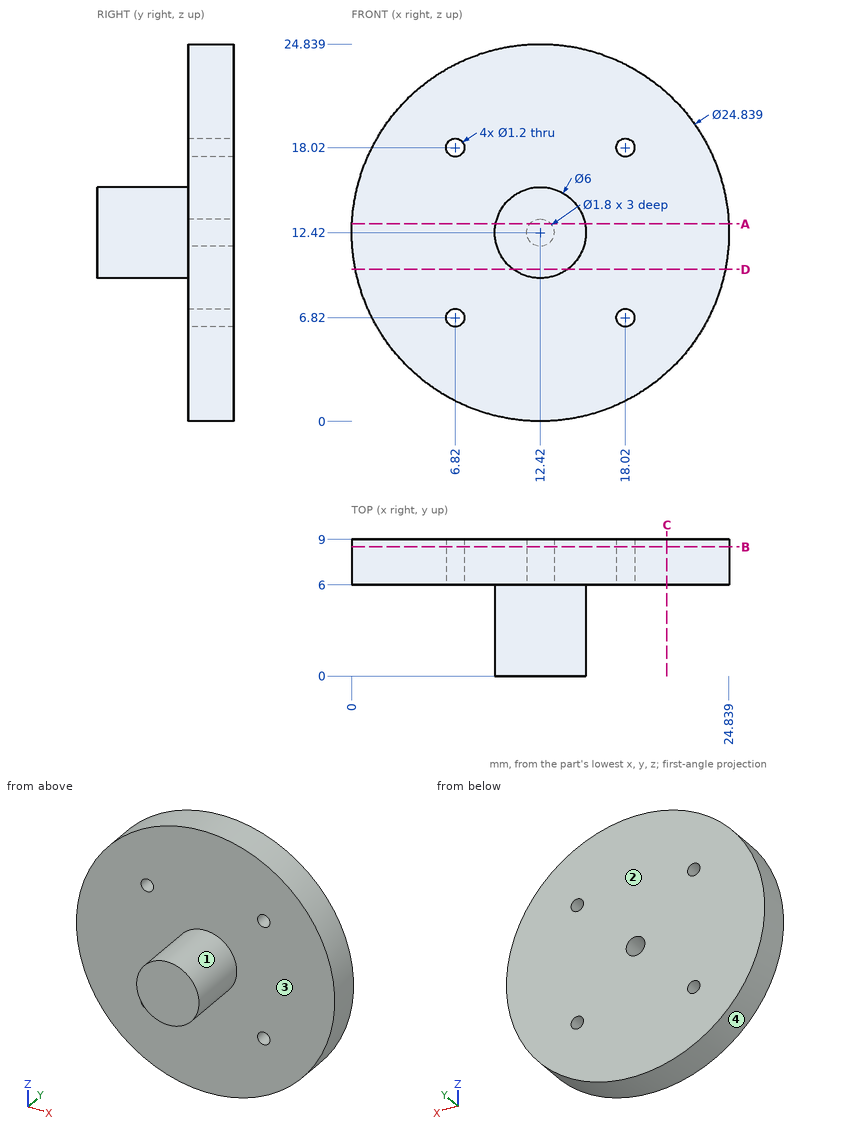
Design review of the part shown in the three views and the two pictorial views. Dimensions are in mm from the part's minimum x, y and z. A direction names the side the tool comes from. Round coordinates to 2 decimals unless told otherwise and drop trailing zeros. Loops run counter-clockwise (first coordinate to the right, second up) from the corner with the lowest first, then second, coordinate; pieces in that order, holes last.
1) The part is to be moulded in two halves that separate along Z. For the marked faces 3 and 4, say which applies: pulls with the +Z half, pulls with the -Z half, needs draft (parallel to the pull), parting line crosses it, or undercut.
Values follow:
face 3: needs draft
face 4: parting line crosses it
2) Consider section D-D on z = 10. State the section outline as (x, y) points.
Values follow:
outline: (0.24, 6) - (10.65, 6) - (10.65, 0) - (14.19, 0) - (14.19, 6) - (24.6, 6) - (24.6, 9) - (0.24, 9) - close
3) Consider section C-C on x = 20.75. State the section outline as (y, z) points.
Values follow:
outline: (6, 3.21) - (9, 3.21) - (9, 21.63) - (6, 21.63) - close
4) Consider section A-A on z = 13. State the section outline as (x, y) points (1 decimal).
Values follow:
outline: (0, 6) - (9.5, 6) - (9.5, 0) - (15.4, 0) - (15.4, 6) - (24.8, 6) - (24.8, 9) - (13.1, 9) - (13.1, 6) - (11.7, 6) - (11.7, 9) - (0, 9) - close
5) Tool access review of the marked faces 1 and 2: name each direction out of +Z, -Z, +X, -X, +Y, -Y from which nothing blocks a thin tool from reaching the whole face with its end or side.
Values follow:
face 1: -Y
face 2: +Z, -Z, +X, -X, +Y
6) Wall thickness on line 1 along Y through (x, z) = (17, 1.75); line 2 along Z through (x, y) = (12.5, 5.75); line 3 along X through (y, z) = (2.25, 12.25) (1 decimal): over which ranges is each line inside the solid? List them lowest first.
Values follow:
line 1: y = 6 to 9
line 2: z = 9.42 to 15.42
line 3: x = 9.4 to 15.4
7) Clearance check with flat-ended pins moving along their axes: P1, Ø1, axis at x = 6.82, z = 18.02, coming from the +Y side; P2, Ø6, axis at x = 15, z = 20, coming from the -Y side; P3, Ø3, axis at x = 10, y = 1, coming from the +Z side (1 decimal); P4, Ø4, axis at x = 15, y = 7, coming from the -Z side. State where each tip first meets the part, or that it passes through.
Values follow:
P1: passes through
P2: stops at y = 6
P3: stops at z = 15.3
P4: stops at z = 0.01
8) Consider section B-B on y = 8.5. State the section outline as (x, z) points.
Values follow:
outline: circle Ø24.84 at (12.42, 12.42); hole circle Ø1.2 at (6.82, 6.82); hole circle Ø1.2 at (6.82, 18.02); hole circle Ø1.8 at (12.42, 12.42); hole circle Ø1.2 at (18.02, 6.82); hole circle Ø1.2 at (18.02, 18.02)
